Check sheet for the modelled part. Datum: model origin and axes. Units: mm. A direction names the side the tool comes from. Give positions to 0.01 mm unless a question says otherwise; leave off trailing zeros. Loops run counter-clockwise (first coordinate to the right, second up) from the corner with the lowest first, then second, coordinate; pieces in that order, holes last. Notation, with made-up numbers: (21, 15) -> (57, 15) arc R30 cw to (57, 53) -> close; hole circle Ø4 at (-34.75, -18.75). An arc over 180 degrees is marked (long way). Answer as CSV lines item,"result". Start each with the question number.
(1) Release check for a two-part mould opening along Z. For faces 1 (the face through (-15.57, 1.63, -13.24)), 2 (the face through (-1, -1, -7)), 3 (the face through (-7, 0, 0)) record: pulls with the +Z half, pulls with the -Z half, needs draft (parallel to the pull), parting line crosses it, or undercut.
(2) Material ranges on line 1 (Y direction, x = -13.5, z = -0.5); line 2 (Z direction, x = -8.75, y = 0.2); line 3 (X direction, y = 1.3, z = -10), recorded low to high. Write a range as from..to.
(3) Section check B-B on x = -5.25. Enter the section's corners in (y, z).
(4) Gauge pin test, flat ends, axial feed: pin 1 Ø0.5 at (y, z) = (0, -7) entering from -X; pin 2 Ø1.7 at (y, z) = (-1.5, -9.5) entering from -X; pin 3 Ø2 at (y, z) = (-1, -6) entering from +X. Record the tip position at first contact, or that the pin passes through.
(5) Section check C-C on y = 0.2. Enter the section's corners in (x, z).
(6) Section check A-A on z = -6. Enter the section's corners in (x, y), plus the area to 3 significant figures.
(7) Access from +Z, -Z, +X, -X, +Y, -Y to the whole of each face (thin tool, end or side, straight path). Record for faces 4 (the face through (-2, -0.5, -7)), 5 (the face through (-8, 0, -12.5)), 6 (the face through (-2, 0.5, -7)), 7 (the face through (-4, 0, -3)), 8 (the face through (0, 1, -7)).
(8) Section check D-D on x = -13.5. Enter the section's corners in (y, z).
from build123d import *

# Parameters (mm, degrees)
SKETCH5_R           = 1.15
SKETCH5_R_2         = 0.749999784
BASE_EXTRUDE_DEPTH  = 14.000000432
SKETCH9_OUTSIDE_W   = 24.639
SKETCH9_OUTSIDE_H   = 20.632
CUT_EXTRUDE2_DEPTH  = 37.000000432
BOSS_EXTRUDE1_DEPTH = 1.000000047


with BuildPart() as part:
    # Sketch5 → Base-Extrude (new body)
    with BuildSketch(Plane.XY):
        with BuildLine():
            Line((-14.650000216, 1.992481203), (-2.16e-07, 2.000000047))
            ThreePointArc((-2.16e-07, 2.000000047), (2.000000047, 1.08e-07), (0, -2.000000047))
            Line((0, -2.000000047), (-15.999999829, -2.000000047))
            Line((-15.999999829, -2.000000047), (-15.999999829, 0.500000071))
            ThreePointArc((-15.999999829, 0.500000071), (-15.656001468, 1.545642629), (-14.650000216, 1.992481203))
        make_face()
        with Locations((-13.500000216, 4.7e-08)):
            Circle(SKETCH5_R, mode=Mode.SUBTRACT)
        Circle(SKETCH5_R_2, mode=Mode.SUBTRACT)
    extrude(amount=-BASE_EXTRUDE_DEPTH)

    # Sketch9 outside → Cut-Extrude2 (cut)
    with BuildSketch(Plane(origin=(0, 17.539650086, 0), x_dir=(-1, 0, 0), z_dir=(0, 1, 0))):
        with Locations((7.0035, -7)):
            Rectangle(SKETCH9_OUTSIDE_W, SKETCH9_OUTSIDE_H)
        Polygon((5.500000203, -12.500000186), (15.999999829, -12.500000186), (15.999999829, -14.000000432), (-1.999999397, -14.000000432), (-1.999999397, -12.500000186), (0, -12.500000186), (0, -1.500000246), (-1.999999397, -1.500000246), (-1.999999397, 0), (15.999999829, 0), (15.999999829, -1.500000246), (5.500000203, -1.500000246), (1.000000164, -1.500000246), (1.000000164, -12.500000186), align=None, mode=Mode.SUBTRACT)
    extrude(amount=-CUT_EXTRUDE2_DEPTH, mode=Mode.SUBTRACT)

    # Sketch10 → Boss-Extrude1 (add)
    with BuildSketch(Plane(origin=(-42.928367292, 0.500000071, -4.00000019), x_dir=(-1, 0, 0), z_dir=(0, 1, 0))):
        Polygon((-37.428367089, 2.499999944), (-39.928367266, 0), (-39.928367266, -6.000000052), (-37.428367089, -8.499999996), (-41.928367128, -8.499999996), (-41.928367128, 2.499999944), align=None)
    extrude(amount=-BOSS_EXTRUDE1_DEPTH)


solid = part.part
Working result:
1,face 1,"needs draft"
1,face 2,"undercut"
1,face 3,"pulls with the +Z half"
2,line 1,"y = -2..-1.15, 1.15..1.99"
2,line 2,"z = -14..-12.5, -1.5..0"
2,line 3,"x = -1..0"
3,outline,"(-2, -14) -> (2, -14) -> (2, -12.5) -> (0.5, -12.5) -> (0.5, -12.25) -> (-0.5, -12.25) -> (-0.5, -12.5) -> (-2, -12.5) -> close; (-2, -1.5) -> (-0.5, -1.5) -> (-0.5, -1.75) -> (0.5, -1.75) -> (0.5, -1.5) -> (2, -1.5) -> (2, 0) -> (-2, 0) -> close"
4,pin 1,"stops at x = -3"
4,pin 2,"stops at x = -1"
4,pin 3,"stops at x = 0"
5,outline,"(-16, -14) -> (-14.63, -14) -> (-14.63, -12.5) -> (-16, -12.5) -> close; (-16, -1.5) -> (-14.63, -1.5) -> (-14.63, 0) -> (-16, 0) -> close; (-12.37, -14) -> (-0.72, -14) -> (-0.72, 0) -> (-12.37, 0) -> (-12.37, -1.5) -> (-5.5, -1.5) -> (-3, -4) -> (-3, -10) -> (-5.5, -12.5) -> (-12.37, -12.5) -> close; (0.72, -14) -> (1.99, -14) -> (1.99, -12.5) -> (0.72, -12.5) -> close; (0.72, -1.5) -> (1.99, -1.5) -> (1.99, 0) -> (0.72, 0) -> close"
6,outline,"(-3, -0.5) -> (-1, -0.5) -> (-1, -2) -> (0, -2) -> (0, -0.75) arc R0.75 cw to (0, 0.75) -> (0, 2) -> (-1, 2) -> (-1, 0.5) -> (-3, 0.5) -> close"
6,area,"5.12 mm^2"
7,face 4,"-X, -Y"
7,face 5,"-X"
7,face 6,"-X, +Y"
7,face 7,"-X, +Y, -Y"
7,face 8,"+X, +Y, -Y"
8,outline,"(-2, -14) -> (-1.15, -14) -> (-1.15, -12.5) -> (-2, -12.5) -> close; (-2, -1.5) -> (-1.15, -1.5) -> (-1.15, 0) -> (-2, 0) -> close; (1.15, -14) -> (1.99, -14) -> (1.99, -12.5) -> (1.15, -12.5) -> close; (1.15, -1.5) -> (1.99, -1.5) -> (1.99, 0) -> (1.15, 0) -> close"
